Autodesk Inventor part; units mm, degrees
ref_plane "Work Plane2" through (0, 0, 5) normal (0, 0, 1) x (1, 0, 0)
ref_plane "Work Plane8" through (0, 0, 0) normal (0.9510565, 0.309017, 0) x (0, 0, 1)
ref_plane "Work Plane9" through (0, 0, 0) normal (1, 0, 0) x (0, 1, 0)
sketch "Sketch1" plane through (0, 0, 0) normal (0, 0, 1) x (1, 0, 0)
  circle A0 centre (0, 0) radius 15
  dimension "d0" = 30
extrude "Extrusion1" add sketch "Sketch1" along normal blind 10
ref_plane "Work Plane2" through (0, 0, 5) normal (0, 0, 1) x (1, 0, 0)
sketch "Sketch2" plane through (0, 0, 0) normal (0, 0, -1) x (-1, 0, 0)
  circle A0 centre (0, 0) radius 15
  circle A1 centre (0, 0) radius 12.5
  dimension "d3" = 25
surface extrude "Pitch Diameter" sketch "Sketch2" against normal through all shown no curves A1
ref_plane "Work Plane8" through (0, 0, 0) normal (0.9510565, 0.309017, 0) x (0, 0, 1)
ref_plane "Work Plane9" through (0, 0, 0) normal (1, 0, 0) x (0, 1, 0)
spur gear teeth "Spur Gear" teeth 10 pitch diameter 25 tip diameter 30 root diameter 18.75 face width 10 start plane through (0, 0, 0) normal (0, 0, -1) x (-1, 0, 0)
equation "\"d0\" = da_da"
equation "\"d1\" = da_b"
equation "\"d3\" = da_d"
properties part number "Spur Gear1" material "Steel"
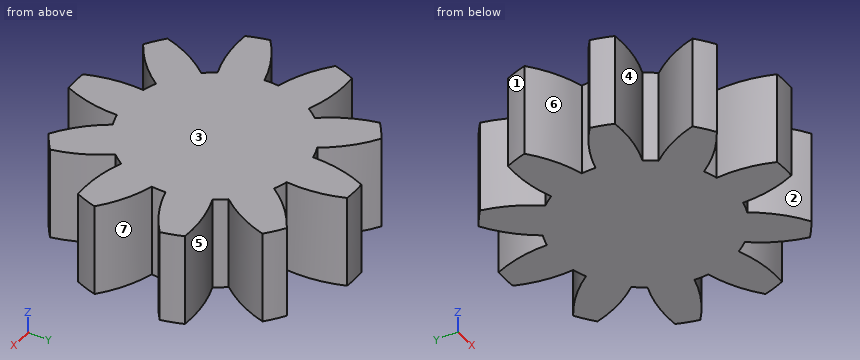
Could you check a few things on this model? Use its own coordinates, in mm. Face numbers are marked on the shaded views. A direction names the side the tool comes from. Coordinates: 2 decimals unless noted, no trailing zeros. Write each loop counter-clockwise with the first axis right and the second up, starting at its lowest first coordinate (ties: lowest second). Pieces come first, ordered by that corner, then holes. Notation, with made-up numbers: (-21, -1.5) -> (31, -1.5) arc R25 cw to (31, 13.5) -> close; hole circle Ø1 at (28, -3). An arc over 180 degrees is marked (long way). Write item = value, one per line. Start each with the question number.
(1) Will these pins go through, and if not, where does the flat tip stop? pin 1 (1.5 mm diameter, centred on x = -11, z = 7.5, fed in from -Y); pin 2 (2 mm diameter, centred on y = -10.5, z = 1, fed in from -X); pin 3 (1.5 mm diameter, centred on x = 6, z = 6.5, fed in from +Y).
(2) I want a section at A-A (x = -11.75). Please give me the cut outline in (y, z), plus the area to 3 significant figures.
(3) I need wall thicknesses on line 1 (X direction, y = 11.5, z = 0.75); line 2 (X direction, y = -10, z = 6); line 3 (Y direction, x = -11.75, z = 9.25). Which ranges of each line are inside material? Lowest first, please. Write a range as [from, to].
(4) We'd pull the mould along Y, two halves only. Please class the marked faces 1, 2, 3 and 4: released by +Y, released by -Y, zero draft, split by the parting line, or undercut.
(5) I want a section at C-C (x = 5.25). Please give me the cut outline in (y, z), plus the area to 3 significant figures.
(6) Which directions (+Z, -Z, +X, -X, +Y, -Y) give clear straight access to the entire face, cutting with the end or side of a thin tool? Please do the marked faces 5, 6 and 7.
(7) I want a section at B-B (y = -8). Please give me the cut outline in (x, z), plus the area to 3 significant figures.
Result set:
q1.pin_1 = -5.74
q1.pin_2 = -9.74
q1.pin_3 = 12.04
q2.outline = (-5.74, 0) -> (-1.64, 0) -> (-1.64, 10) -> (-5.74, 10) -> close; (1.64, 0) -> (5.74, 0) -> (5.74, 10) -> (1.64, 10) -> close
q2.area = 81.8 mm2
q3.line_1 = [-9.63, -6.08], [-2.09, 2.09], [6.08, 9.63]
q3.line_2 = [-9.32, -4.59], [-2.2, 2.2], [4.59, 9.32]
q3.line_3 = [-5.74, -1.64], [1.64, 5.74]
q4.face_1 = released by +Y
q4.face_2 = released by -Y
q4.face_3 = zero draft
q4.face_4 = undercut
q5.outline = (-10.72, 0) -> (10.72, 0) -> (10.72, 10) -> (-10.72, 10) -> close
q5.area = 214 mm2
q6.face_5 = +Z, -Z
q6.face_6 = +Z, -Z, -X
q6.face_7 = +Z, -Z, +X
q7.outline = (-8.41, 0) -> (8.41, 0) -> (8.41, 10) -> (-8.41, 10) -> close
q7.area = 168 mm2
